Check sheet for the modelled part. Datum: model origin and axes. Units: mm. A direction names the side the tool comes from. Give positions to 0.01 mm unless a question says otherwise; leave off trailing zeros. Loops run counter-clockwise (first coordinate to the right, second up) from the corner with the lowest first, then second, coordinate; pieces in that order, holes last. Notation, with made-up numbers: (-33, 32) - (3, 32) arc R4 ccw to (3, 38) - close; hole circle Ø5 at (60, 4). An arc over 180 degrees is marked (long way). Use one line per item in the form item = value.
from build123d import *

# Parameters (mm, degrees)
PAD_DEPTH       = 107
SKETCH001_W     = 101
SKETCH001_H     = 42
POCKET_DEPTH    = 42.3
SKETCH002_W     = 101
SKETCH002_H     = 56
POCKET001_DEPTH = 34.14
SKETCH003_W     = 101
SKETCH003_H     = 83.7
POCKET002_DEPTH = 15.16
SKETCH004_W     = 11.6
SKETCH004_H     = 91.85
POCKET003_DEPTH = 87.701
POCKET004_DEPTH = 5


with BuildPart() as part:
    # Sketch → Pad (new body)
    with BuildSketch(Plane.YZ):
        with BuildLine():
            Line((0, 0), (0, -87.7))
            Line((0, -87.7), (16.54, -87.7))
            Line((16.54, -87.7), (16.54, -73.85))
            Line((16.54, -73.85), (35.54, -73.85))
            Line((35.54, -73.85), (35.54, -66.85))
            Line((35.54, -66.85), (44.54, -66.85))
            ThreePointArc((44.54, -66.85), (49.84, -43.85), (44.54, -20.85))
            Line((44.54, -20.85), (35.54, -20.85))
            Line((35.54, -20.85), (35.54, -13.85))
            Line((35.54, -13.85), (16.54, -13.85))
            Line((16.54, -13.85), (16.54, 0))
            Line((16.54, 0), (0, 0))
        make_face()
    extrude(amount=PAD_DEPTH)

    # Sketch001 → Pocket (cut)
    with BuildSketch(Plane.XZ):
        with Locations((53.5, -43.85)):
            Rectangle(SKETCH001_W, SKETCH001_H)
    extrude(amount=-POCKET_DEPTH, mode=Mode.SUBTRACT)

    # Sketch002 → Pocket001 (cut)
    with BuildSketch(Plane.XZ):
        with Locations((53.5, -43.85)):
            Rectangle(SKETCH002_W, SKETCH002_H)
    extrude(amount=-POCKET001_DEPTH, mode=Mode.SUBTRACT)

    # Sketch003 → Pocket002 (cut)
    with BuildSketch(Plane.XZ):
        with Locations((53.5, -43.85)):
            Rectangle(SKETCH003_W, SKETCH003_H)
    extrude(amount=-POCKET002_DEPTH, mode=Mode.SUBTRACT)

    # Sketch004 (on Face5 of Pocket002) → Pocket003 (cut, through all)
    with BuildSketch(Plane.YX.offset(87.7)):
        with Locations((5.8, 53.5)):
            Rectangle(SKETCH004_W, SKETCH004_H)
    extrude(amount=-POCKET003_DEPTH, mode=Mode.SUBTRACT)

    # Sketch005 (on Face10 of Pocket003) → Pocket004 (cut)
    with BuildSketch(Plane.ZX.offset(16.54)):
        with BuildLine():
            ThreePointArc((-78.55, 96), (-81.15, 98.6), (-83.75, 96))
            Line((-83.75, 96), (-83.75, 11))
            ThreePointArc((-83.75, 11), (-81.15, 8.4), (-78.55, 11))
            Line((-78.55, 96), (-78.55, 11))
        make_face()
        with BuildLine():
            ThreePointArc((-3.95, 96), (-6.55, 98.6), (-9.15, 96))
            Line((-9.15, 96), (-9.15, 11))
            ThreePointArc((-9.15, 11), (-6.55, 8.4), (-3.95, 11))
            Line((-3.95, 96), (-3.95, 11))
        make_face()
    extrude(amount=-POCKET004_DEPTH, mode=Mode.SUBTRACT)


solid = part.part
Item 1: Thickness scan on L1, parallel to X at y = 26.5, z = -48; L2, parallel to Z at x = 79, y = 22; L3, parallel to Z at x = 11.5, y = 34.5. Record the ranges inside material, lowest first.
Answer block:
L1 = 0 to 3, 104 to 107
L2 = -73.85 to -71.85, -15.85 to -13.85
L3 = -73.85 to -64.85, -22.85 to -13.85
Item 2: Section check B-B on y = 39.5. Record the boundary of the cut face in (x, z), then the cut area to 3 significant figures.
Answer block:
outline = (0, -66.85) - (107, -66.85) - (107, -20.85) - (0, -20.85) - close; hole (3, -64.85) - (104, -64.85) - (104, -22.85) - (3, -22.85) - close
area = 680 mm2
Item 3: Section check C-C on x = 18. Give the number of separate pieces and of enclosed holes in the cut face, then the cut area to 3 significant figures.
Answer block:
separate_pieces = 3
enclosed_holes = 0
area = 434 mm2
Item 4: Mould release check, pull along Z, two halves, no side actions. Record for faces 1 (the face through (53, 40, -66.85)), 2 (the face through (53, 16.54, -10)), 3 (the face through (53, 15.16, -10)), 4 (the face through (8.4, 15.9, -81.2)): released by +Z, released by -Z, zero draft, split by the parting line, or undercut.
Answer block:
face_1 = released by -Z
face_2 = zero draft
face_3 = undercut
face_4 = undercut
Item 5: Section check A-A on z = -6.55. Record the boundary of the cut face in (x, y), then the cut area to 3 significant figures.
Answer block:
outline = (0, 0) - (3, 0) - (3, 15.16) - (8.4, 15.16) - (8.4, 16.54) - (0, 16.54) - close; (98.6, 15.16) - (104, 15.16) - (104, 0) - (107, 0) - (107, 16.54) - (98.6, 16.54) - close
area = 114 mm2
Item 6: Section check D-D on y = 8. Record the boundary of the cut face in (x, z) (3 decimals).
Answer block:
outline = (0, -87.7) - (7.575, -87.7) - (7.575, -85.7) - (3, -85.7) - (3, -2) - (7.575, -2) - (7.575, 0) - (0, 0) - close; (99.425, -87.7) - (107, -87.7) - (107, 0) - (99.425, 0) - (99.425, -2) - (104, -2) - (104, -85.7) - (99.425, -85.7) - close
Item 7: Gauge pin test, flat ends, axial feed: P1, Ø10, axis at x = 54.5, y = 25.5, coming from the +Z side; P2, Ø4.5, axis at x = 51, y = 39, coming from the -Z side; P3, Ø1.6, axis at x = 75, z = -0.5, coming from the -Y side. Record the tip position at first contact, or that the pin passes through.
Answer block:
P1 = -13.85
P2 = -66.85
P3 = 11.6
Item 8: Access from +Z, -Z, +X, -X, +Y, -Y to the whole of each face (thin tool, end or side, straight path). Record for faces 5 (the face through (53, 35.54, -70)), 6 (the face through (53, 38, -64.85)), 7 (the face through (53, 12, -87.7)).
Answer block:
face_5 = -Z, +X, -X, +Y
face_6 = -Y
face_7 = -Z, +X, -X, +Y, -Y
